Geometry: final body of the model. Coordinates: model frame, mm. Face numbers are marked on the shaded views. A direction names the side the tool comes from. Give positions to 0.01 mm unless a question says otherwise; leave off trailing zeros. Order: outer loops, then holes, each group sorted by start corner. A loop starts at its lowest first (then second) coordinate and runs counter-clockwise, first axis right, second up. Notation, with made-up numbers: (49.5, -36.75) - (80.5, -36.75) arc R31 ccw to (80.5, -9.75) - close; hole circle Ø2 at (31, 67). An arc over 180 degrees is marked (long way). One line per item, written item: value.
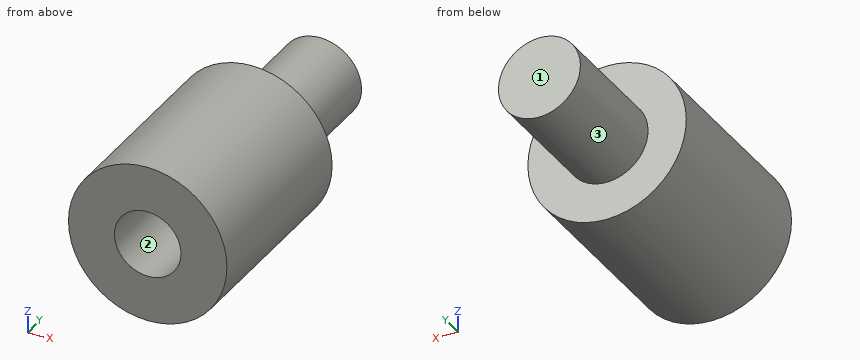
```python
from build123d import *

# Parameters (mm, degrees)
OD_BASE_R           = 2.9
STANDOFF_BASE_DEPTH = 7
OD_POST_MOUNT_R     = 1.5
STANDOFF_POST_DEPTH = 4.5
ID_POST_MOUNT_R     = 1.2195
POST_MOUNT_DEPTH    = 3


with BuildPart() as part:
    # OD_base → standoff_base (new body)
    with BuildSketch(Plane(origin=(0, 0, 0), x_dir=(1, 0, 0), z_dir=(0, 1, 0))):
        with Locations(Location((0, 0, 0), (0, 0, 270))):
            Circle(OD_BASE_R)
    extrude(amount=STANDOFF_BASE_DEPTH)

    # OD_post_mount → standoff_post (add)
    with BuildSketch(Plane(origin=(0, 7, 0), x_dir=(1, 0, 0), z_dir=(0, 1, 0))):
        with Locations(Location((0, 0, 0), (0, 0, 270))):
            Circle(OD_POST_MOUNT_R)
    extrude(amount=STANDOFF_POST_DEPTH)

    # ID_post_mount → post_mount (cut)
    with BuildSketch(Plane.XZ):
        with Locations(Location((0, 0, 0), (0, 0, 270))):
            Circle(ID_POST_MOUNT_R)
    extrude(amount=-POST_MOUNT_DEPTH, mode=Mode.SUBTRACT)


solid = part.part
```
1) Section A-A, the plane x = 0. Return loops of the section in (y, z), then the cut area to 3 significant figures.
Answers below:
outline: (0, -2.9) - (7, -2.9) - (7, -1.5) - (11.5, -1.5) - (11.5, 1.5) - (7, 1.5) - (7, 2.9) - (0, 2.9) - (0, 1.22) - (3, 1.22) - (3, -1.22) - (0, -1.22) - close
area: 46.8 mm^2
2) Section C-C, the plane y = 1.5. Return loops of the section in (x, z).
Answers below:
outline: circle Ø5.8 at (0, 0); hole circle Ø2.44 at (0, 0)
3) Set-up query: the marked faces 1, 2 and 3. Return all of +Z, -Z, +X, -X, +Y, -Y with unobstructed straight access to the full face (end or side cutting, diameter ignored); none if empty.
Answers below:
face 1: +Z, -Z, +X, -X, +Y
face 2: -Y
face 3: +Y
4) First-contact query: pin 1 (3 mm diameter, centred on y = 3.5, z = 2.5, fed in from -X); pin 2 (3 mm diameter, centred on y = 10, z = 1, fed in from +X). Flat tips, straight axial feed; report the tip coordinate or a pass-through.
Answers below:
pin 1: x = -2.72
pin 2: x = 1.5
5) Material intervals for line 1 along X through (y, z) = (0.7, 0); line 2 along Y through (x, z) = (0.25, -1.85); line 3 along Y through (x, z) = (-0.85, 0.8), sorted ascending.
Answers below:
line 1: -2.9 to -1.22, 1.22 to 2.9
line 2: 0 to 7
line 3: 3 to 11.5
6) Section D-D, the plane y = 6.75. Return loops of the section in (x, z), then the cut area to 3 significant figures.
Answers below:
outline: circle Ø5.8 at (0, 0)
area: 26.4 mm^2
7) Section B-B, the plane z = 0. Return loops of the section in (x, y), then the cut area to 3 significant figures.
Answers below:
outline: (-2.9, 0) - (-1.22, 0) - (-1.22, 3) - (1.22, 3) - (1.22, 0) - (2.9, 0) - (2.9, 7) - (1.5, 7) - (1.5, 11.5) - (-1.5, 11.5) - (-1.5, 7) - (-2.9, 7) - close
area: 46.8 mm^2
